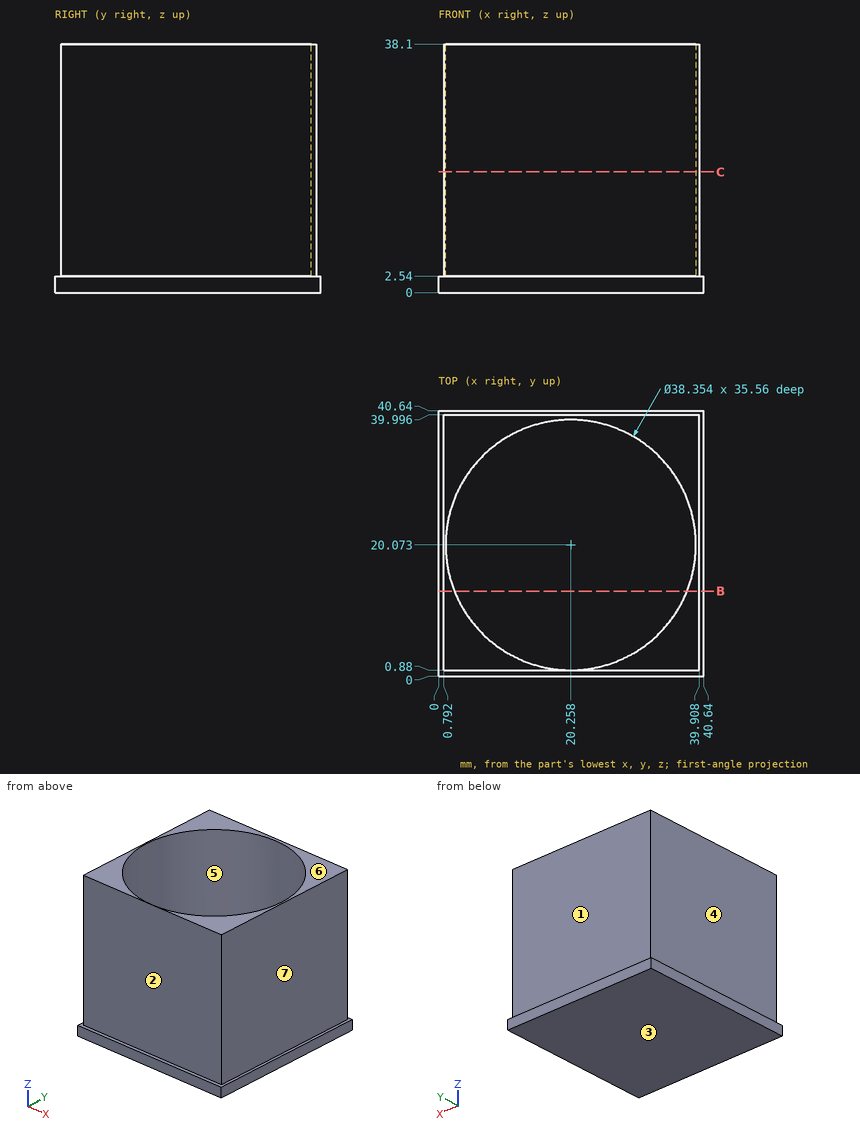
Here's the drawing with two shaded views (mm, measured from the low corner). I have some questions. A direction names the side the tool comes from. Round coordinates to 2 decimals unless told otherwise and drop trailing zeros. Order: outer loops, then holes, each group sorted by start corner. A loop starts at its lowest first (then second) coordinate and runs counter-clockwise, first axis right, second up. Notation, with made-up numbers: M -5,28 L 10,28 A11 ccw 10,32 Z; hole C 6,54 d1. An arc over 180 degrees is marked long. Use CSV: the item, a comma, the result in double quotes.
1) I'm going to push flat-ended pins straight in: P1, Ø10.5, axis at x = 27, z = 16, coming from the -Y side; P2, Ø20.5, axis at x = 25.5, y = 27, coming from the +Z side; P3, Ø10, axis at y = 14, z = 15.5, coming from the -X side. Where does each tip first touch, or does it pass through?
Taken from the geometry:
P1,"y = 0.88"
P2,"z = 2.54"
P3,"x = 0.79"
2) I want a section at B-B (y = 13). List the corners of the cut face in (x, z) for me.
Taken from the geometry:
outline,"M 0,0 L 40.64,0 L 40.64,2.54 L 39.91,2.54 L 39.91,38.1 L 38.08,38.1 L 38.08,2.54 L 2.43,2.54 L 2.43,38.1 L 0.79,38.1 L 0.79,2.54 L 0,2.54 Z"
3) I want a section at C-C (z = 18.5). List the corners of the cut face in (x, y) for me (1 decimal), then the cut area to 3 significant figures.
Taken from the geometry:
outline,"M 0.8,0.9 L 39.9,0.9 L 39.9,40 L 0.8,40 Z; hole C 20.3,20.1 d38.4"
area,"375 mm^2"
4) If we mould it in two halves opening along X, with no side actions, what happens to the marked faces 5, 6 and 7? For each: pulls with the +X half, pulls with the -X half, needs draft (parallel to the pull), parting line crosses it, or undercut.
Taken from the geometry:
face 5,"undercut"
face 6,"needs draft"
face 7,"pulls with the +X half"
5) On a 3-axis mill with a long thin cutter (end or side, diameter ignored), from which of +Z, -Z, +X, -X, +Y, -Y can I reach the whole of each face in a straight line? I mean the marked faces 1, 2, 3 and 4. Say none if no direction works.
Taken from the geometry:
face 1,"+Z, +X, -X, +Y"
face 2,"+Z, +X, -X, -Y"
face 3,"-Z, +X, -X, +Y, -Y"
face 4,"+Z, -X, +Y, -Y"
6) I need wall thicknesses on line 1 along Z through (x, y) = (14.5, 10.5); line 2 along Y through (x, z) = (25, 10) (1 decimal); line 3 along Y through (x, z) = (35, 15.5) (1 decimal). Which ranges of each line are inside material? Lowest first, please. Write a range as [from, to].
Taken from the geometry:
line 1,"[0, 2.54]"
line 2,"[0.9, 1.5], [38.7, 40]"
line 3,"[0.9, 7.8], [32.3, 40]"
